Here's how the part is built. I have some questions about the finished solid (model axes, mm). Round coordinates to 2 decimals unless told otherwise and drop trailing zeros. Write each loop counter-clockwise with the first axis right and the second up, starting at its lowest first coordinate (ties: lowest second). Pieces come first, ordered by that corner, then holes. Notation, with made-up numbers: (-21.75, 22.25) -> (6.25, 22.25) arc R6 ccw to (6.25, 31.25) -> close; hole circle Ø11 at (38.5, 79.5). An arc over 180 degrees is marked (long way). Put each result on its own line as item: value. Start each with the question number.
1. I need wall thicknesses on probe 1 along X at (y, z) = (1.55, -55); probe 2 along X at (y, z) = (1.7, -78). Which ranges of each line are inside material? Lowest first, please. Write a range as from..to.
2. Suppose I cut it at B-B (x = -55). Please give me the cut outline in (y, z).
3. Suppose I cut it at C-C (y = 0.95). Please give me the cut outline in (x, z), then the cut area to 3 significant figures.
4. Suppose I cut it at A-A (z = -55). Please give me the cut outline in (x, y).
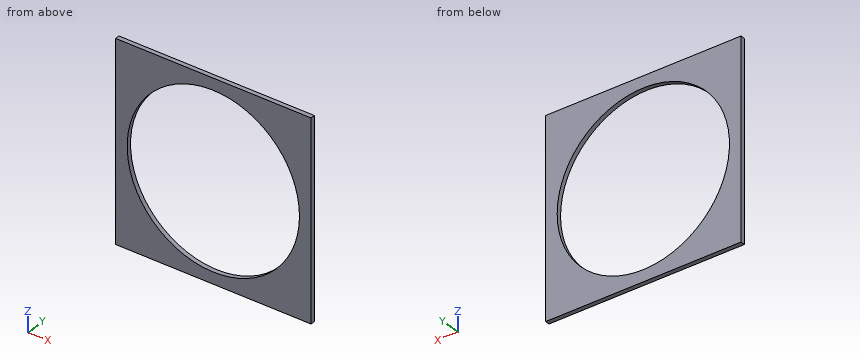
Autodesk Inventor part; units mm, degrees
ref_plane "YZ Plane" through (0, 0, 0) normal (1, 0, 0) x (0, 1, 0)
ref_plane "XZ Plane" through (0, 0, 0) normal (0, 1, 0) x (-1, 0, 0)
ref_plane "XY Plane" through (0, 0, 0) normal (0, 0, 1) x (1, 0, 0)
sketch "Sketch1" plane through (0, 0, 0) normal (0, 1, 0) x (-1, 0, 0)
  line L0 (0, 0) -> (110, 0)
  line L1 (110, 0) -> (110, -110)
  line L2 (110, -110) -> (0, -110)
  line L3 (0, -110) -> (0, 0)
  dimension "d0" = 110
  dimension "d1" = 110
extrude "Extrusion1" add sketch "Sketch1" along normal blind 2.5
sketch "Sketch2" plane through (0, 2.5, 0) normal (0, 1, 0) x (1, 0, 0)
  line L0 (-110, 110) -> (-110, 0)
  line L1 (-110, 0) -> (0, 0)
  circle A0 centre (-55, 55) radius 48.5
extrude "Extrusion2" cut sketch "Sketch2" against normal blind 2.5
properties part number "AdapterRing"
Verdict:
1. probe 1: x = -110..-103.5, -6.5..0
1. probe 2: x = -110..-97.7, -12.3..0
2. outline: (0, -110) -> (2.5, -110) -> (2.5, -103.5) -> (0, -103.5) -> close; (0, -6.5) -> (2.5, -6.5) -> (2.5, 0) -> (0, 0) -> close
3. outline: (-110, -110) -> (0, -110) -> (0, 0) -> (-110, 0) -> close; hole circle Ø97 at (-55, -55)
3. area: 4,710 mm^2
4. outline: (-110, 0) -> (-103.5, 0) -> (-103.5, 2.5) -> (-110, 2.5) -> close; (-6.5, 0) -> (0, 0) -> (0, 2.5) -> (-6.5, 2.5) -> close
